Print and shaded views of the part. All mm, measured from the part's lowest x, y and z. Round coordinates to 2 decimals unless told otherwise and drop trailing zeros. Write each loop counter-clockwise with the first axis right and the second up, starting at its lowest first coordinate (ties: lowest second). Pieces come first, ordered by that corner, then holes. Notation, with made-up numbers: (-28, 67.25) - (-8, 67.25) arc R20 ccw to (-8, 73.25) - close; hole circle Ø10 at (10, 31.25). An arc over 180 degrees is marked (long way). One line per item, written item: value.
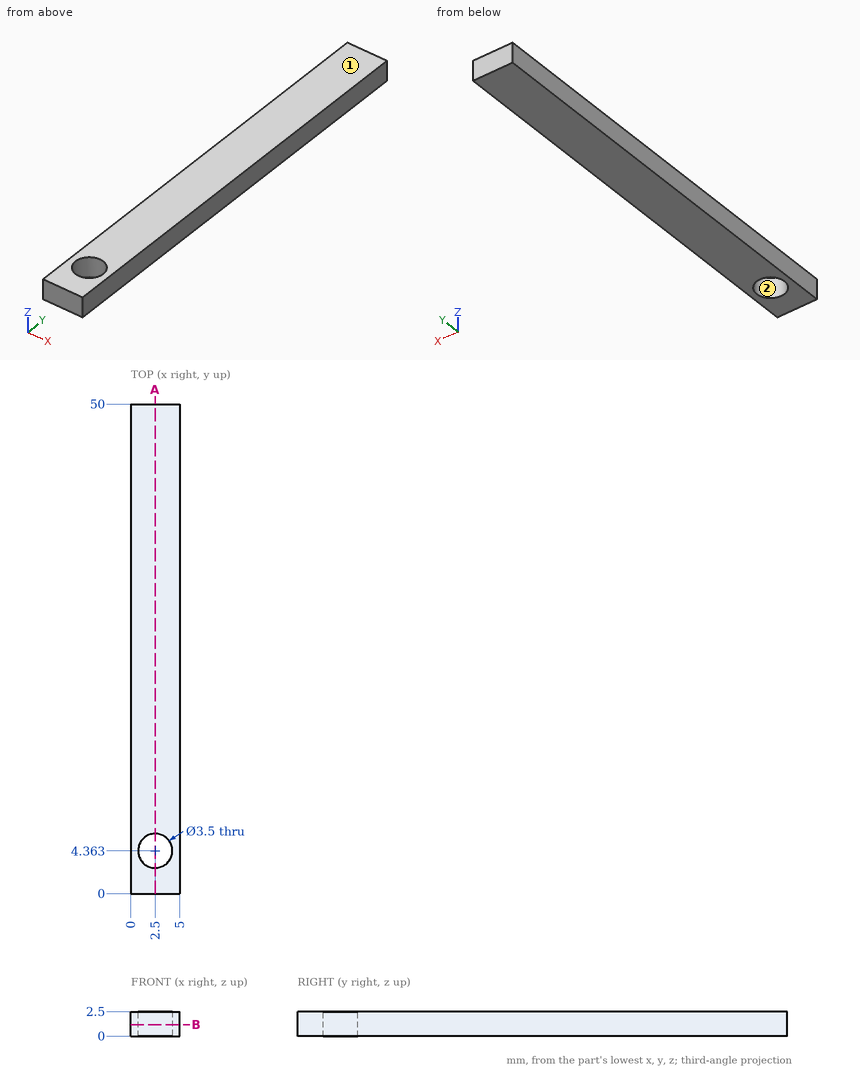
1. Wall check: probe 1 along Y at (x, z) = (2.5, 1.2); probe 2 along X at (y, z) = (4.5, 1.9); probe 3 along Y at (x, z) = (3.8, 0.9) (1 decimal). Give the ranges that are in metal, low to high. Write a range as [from, to].
Report:
probe 1: [0, 2.61], [6.11, 50]
probe 2: [0, 0.76], [4.24, 5]
probe 3: [0, 3.2], [5.5, 50]
2. Band-saw the part on B-B on z = 1.15. Write the cut outline in (x, y).
Report:
outline: (0, 0) - (5, 0) - (5, 50) - (0, 50) - close; hole circle Ø3.5 at (2.5, 4.36)
3. Band-saw the part on A-A on x = 2.5. Write the cut outline in (y, z).
Report:
outline: (0, 0) - (2.61, 0) - (2.61, 2.5) - (0, 2.5) - close; (6.11, 0) - (50, 0) - (50, 2.5) - (6.11, 2.5) - close
4. Mould opens along X. For the marked faces 1 and 2 say: released by +X, released by -X, zero draft, split by the parting line, or undercut.
Report:
face 1: zero draft
face 2: undercut
